Design review of the part built by this model. Coordinates are the model's own, in mm. Face numbers are marked on the shaded views. A direction names the side the tool comes from. Give positions to 0.01 mm unless a question says otherwise; leave off trailing zeros. Order: outer loops, then holes, each group sorted by start corner. A loop starts at its lowest first (then second) coordinate and runs counter-clockwise, first axis right, second up. Notation, with made-up numbers: M 64,80 L 114,80 A7 ccw 114,90 Z; hole C -19.75,26 d1. An arc over 180 degrees is marked long. Put each result on its own line as item: value. Start each with the question number.
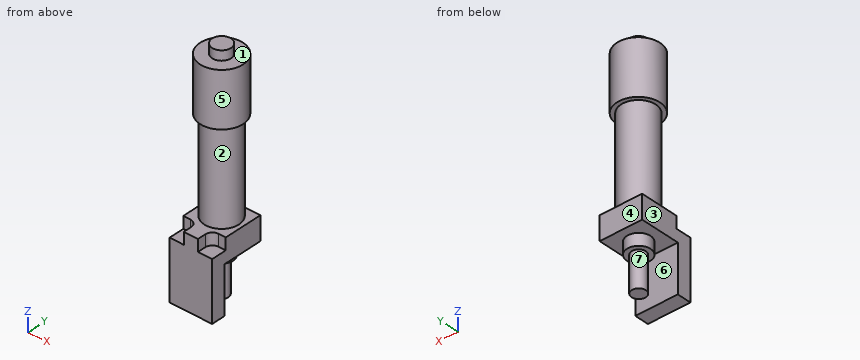
from build123d import *

# Parameters (mm, degrees)
BOSS_EXTRUDE1_DEPTH = 18
CUT_EXTRUDE1_DEPTH  = 5
SKETCH4_R           = 5
BOSS_EXTRUDE2_DEPTH = 5
SKETCH5_R           = 3
BOSS_EXTRUDE3_DEPTH = 15
SKETCH6_R           = 7.35
BOSS_EXTRUDE4_DEPTH = 39.5
SKETCH7_R           = 9.1
BOSS_EXTRUDE5_DEPTH = 23
SKETCH8_R           = 4
BOSS_EXTRUDE6_DEPTH = 4


with BuildPart() as part:
    # Sketch1 → Boss-Extrude1 (new body)
    with BuildSketch(Plane(origin=(0, 0, 0), x_dir=(0, 0, -1), z_dir=(1, 0, 0))):
        Polygon((0, 0), (30, 0), (30, 6), (10, 6), (10, 23), (0, 23), align=None)
    extrude(amount=BOSS_EXTRUDE1_DEPTH)

    # Sketch2 → Cut-Extrude1 (cut)
    with BuildSketch(Plane.XY):
        with BuildLine():
            Line((12, 0), (12, 3.5))
            ThreePointArc((12, 3.5), (12.878679656, 5.621320344), (15, 6.5))
            Line((15, 6.5), (18, 6.5))
            Line((18, 6.5), (18, 0))
            Line((18, 0), (12, 0))
        make_face()
        with BuildLine():
            Line((6, 0), (6, 3.5))
            ThreePointArc((6, 3.5), (5.121320344, 5.621320344), (3, 6.5))
            Line((3, 6.5), (0, 6.5))
            Line((0, 6.5), (0, 0))
            Line((0, 0), (6, 0))
        make_face()
    extrude(amount=-CUT_EXTRUDE1_DEPTH, mode=Mode.SUBTRACT)

    # Sketch4 → Boss-Extrude2 (add)
    with BuildSketch(Plane(origin=(0, 0, -10), x_dir=(-1, 0, 0), z_dir=(0, 0, -1))):
        with Locations(Location((-9, 14.5, 0), (0, 0, 270))):
            Circle(SKETCH4_R)
    extrude(amount=BOSS_EXTRUDE2_DEPTH)

    # Sketch5 → Boss-Extrude3 (add)
    with BuildSketch(Plane(origin=(0, 0, -15), x_dir=(-1, 0, 0), z_dir=(0, 0, -1))):
        with Locations(Location((-9, 14.5, 0), (0, 0, 90))):
            Circle(SKETCH5_R)
    extrude(amount=BOSS_EXTRUDE3_DEPTH)

    # Sketch6 → Boss-Extrude4 (add)
    with BuildSketch(Plane.XY):
        with Locations((9, 14.65)):
            Circle(SKETCH6_R)
    extrude(amount=BOSS_EXTRUDE4_DEPTH)

    # Sketch7 → Boss-Extrude5 (add)
    with BuildSketch(Plane.XY.offset(39.5)):
        with Locations((9, 14.65)):
            Circle(SKETCH7_R)
    extrude(amount=BOSS_EXTRUDE5_DEPTH)

    # Sketch8 → Boss-Extrude6 (add)
    with BuildSketch(Plane.XY.offset(62.5)):
        with Locations((9, 14.65)):
            Circle(SKETCH8_R)
    extrude(amount=BOSS_EXTRUDE6_DEPTH)


solid = part.part
1. Consider section D-D on z = 58. Give the boundary of the cut face in (x, y), then the cut area to 3 significant figures.
2. Consider section B-B on x = 9. Give the boundary of the cut face in (y, z).
3. Consider section C-C on y = 16.25. Give the boundary of the cut face in (x, z).
4. Consider section A-A on z = -20. Give the boundary of the cut face in (x, y), then the cut area to 3 significant figures.
5. The part is to be moulded in two halves that separate along Z. For the marked faces 1, 2 and 3, say which applies: +Z half, -Z half, draft (parallel to the pull), parting line (faces both ways), or undercut.
6. Insertion check: pin 1 (4 mm diameter, centred on x = 14.5, z = -18, fed in from -Y); pin 2 (4 mm diameter, centred on x = 7, y = 3.5, fed in from +Z); pin 3 (6.5 mm diameter, centred on x = 15.5, y = 5, fed in from +Z); pin 4 (3.5 mm diameter, centred on x = 2, z = -2.5, fed in from -Y). Each pin has a flat end and moves straight along its axis. Give the tip position at first contact, or say it passes through.
7. To check wall thickness, follow probe 1 along Z at (x, y) = (15.75, 21.25); probe 2 along Z at (x, y) = (14, 2.75); probe 3 along Y at (x, z) = (8.25, -5.5). State the ranges of each line that lie inside material, in increasing order.
8. Machinability: for the marked faces 4, 5, 6 and 7, which of the approach directions +Z, -Z, +X, -X, +Y, -Y give a long, thin tool a straight path to every point of the face, cutting with its end or side? Answer none if there is none.
Returned:
1. outline: C 9,14.65 d18.2
1. area: 260 mm2
2. outline: M 0,-30 L 6,-30 L 6,-10 L 9.5,-10 L 9.5,-15 L 11.5,-15 L 11.5,-30 L 17.5,-30 L 17.5,-15 L 19.5,-15 L 19.5,-10 L 23,-10 L 23,0 L 22,0 L 22,39.5 L 23.75,39.5 L 23.75,62.5 L 18.65,62.5 L 18.65,66.5 L 10.65,66.5 L 10.65,62.5 L 5.55,62.5 L 5.55,39.5 L 7.3,39.5 L 7.3,0 L 0,0 Z
3. outline: M 0,-10 L 4.32,-10 L 4.32,-15 L 6.56,-15 L 6.56,-30 L 11.44,-30 L 11.44,-15 L 13.68,-15 L 13.68,-10 L 18,-10 L 18,0 L 16.17,0 L 16.17,39.5 L 17.96,39.5 L 17.96,62.5 L 12.67,62.5 L 12.67,66.5 L 5.33,66.5 L 5.33,62.5 L 0.04,62.5 L 0.04,39.5 L 1.83,39.5 L 1.83,0 L 0,0 Z
4. outline: M 0,0 L 18,0 L 18,6 L 0,6 Z; C 9,14.5 d6
4. area: 136 mm2
5. face 1: +Z half
5. face 2: undercut
5. face 3: draft
6. pin 1: stops at y = 0
6. pin 2: stops at z = 0
6. pin 3: stops at z = 62.5
6. pin 4: stops at y = 6.4
7. probe 1: z = -10 to 0
7. probe 2: z = -30 to -5
7. probe 3: y = 0 to 23
8. face 4: -Z, +X, -X, +Y
8. face 5: +Z
8. face 6: -Z, +X, -X
8. face 7: -Z
